```python
from build123d import *

# Parameters (mm, degrees)
ESQUISSE1_W             = 55
ESQUISSE1_H             = 55
BOSS_EXTRU_1_DEPTH      = 5
ESQUISSE2_W             = 30
ESQUISSE2_H             = 15
BOSS_EXTRU_2_DEPTH      = 60
CONG_2_R                = 5
CONG_3_R                = 5
CONG_4_R                = 5
CONG_5_R                = 5
ENL_V_MAT_EXTRU_1_REACH = 7
ESQUISSE3_R             = 1
ESQUISSE4_R             = 0.5
ENL_V_MAT_EXTRU_2_DEPTH = 2


with BuildPart() as part:
    # Esquisse1 → Boss.-Extru.1 (new body)
    with BuildSketch(Plane.XY):
        Rectangle(ESQUISSE1_W, ESQUISSE1_H)
    extrude(amount=BOSS_EXTRU_1_DEPTH)

    # Esquisse2 → Boss.-Extru.2 (add)
    with BuildSketch(Plane.XY.offset(5)):
        Rectangle(ESQUISSE2_W, ESQUISSE2_H)
    extrude(amount=BOSS_EXTRU_2_DEPTH)

    # Congé2
    cong_2_edges = [part.edges().sort_by_distance(p)[0] for p in [
        (-15, -7.5, 35),
    ]]
    fillet(cong_2_edges, radius=CONG_2_R)

    # Congé3
    cong_3_edges = [part.edges().sort_by_distance(p)[0] for p in [
        (15, 7.5, 35),
    ]]
    fillet(cong_3_edges, radius=CONG_3_R)

    # Congé4
    cong_4_edges = [part.edges().sort_by_distance(p)[0] for p in [
        (15, -7.5, 35),
    ]]
    fillet(cong_4_edges, radius=CONG_4_R)

    # Congé5
    cong_5_edges = [part.edges().sort_by_distance(p)[0] for p in [
        (-15, 7.5, 35),
    ]]
    fillet(cong_5_edges, radius=CONG_5_R)

    # Esquisse3 → Enlèv. mat.-Extru.1 (cut, up to next)
    with BuildSketch(Plane.XY.offset(5), mode=Mode.PRIVATE) as enl_v_mat_extru_1_sk1:
        with Locations((17.5, 17.5)):
            Circle(ESQUISSE3_R)
    enl_v_mat_extru_1_tool1 = extrude(enl_v_mat_extru_1_sk1.sketch, amount=-ENL_V_MAT_EXTRU_1_REACH, mode=Mode.PRIVATE) & part.part
    add(enl_v_mat_extru_1_tool1.solids().sort_by_distance((17.5, 17.5, 5))[0], mode=Mode.SUBTRACT)
    # Esquisse3 → Enlèv. mat.-Extru.1 (cut, up to next)
    with BuildSketch(Plane.XY.offset(5), mode=Mode.PRIVATE) as enl_v_mat_extru_1_sk2:
        with Locations((-17.5, 17.5)):
            Circle(ESQUISSE3_R)
    enl_v_mat_extru_1_tool2 = extrude(enl_v_mat_extru_1_sk2.sketch, amount=-ENL_V_MAT_EXTRU_1_REACH, mode=Mode.PRIVATE) & part.part
    add(enl_v_mat_extru_1_tool2.solids().sort_by_distance((-17.5, 17.5, 5))[0], mode=Mode.SUBTRACT)
    # Esquisse3 → Enlèv. mat.-Extru.1 (cut, up to next)
    with BuildSketch(Plane.XY.offset(5), mode=Mode.PRIVATE) as enl_v_mat_extru_1_sk3:
        with Locations((-17.5, -17.5)):
            Circle(ESQUISSE3_R)
    enl_v_mat_extru_1_tool3 = extrude(enl_v_mat_extru_1_sk3.sketch, amount=-ENL_V_MAT_EXTRU_1_REACH, mode=Mode.PRIVATE) & part.part
    add(enl_v_mat_extru_1_tool3.solids().sort_by_distance((-17.5, -17.5, 5))[0], mode=Mode.SUBTRACT)
    # Esquisse3 → Enlèv. mat.-Extru.1 (cut, up to next)
    with BuildSketch(Plane.XY.offset(5), mode=Mode.PRIVATE) as enl_v_mat_extru_1_sk4:
        with Locations((17.5, -17.5)):
            Circle(ESQUISSE3_R)
    enl_v_mat_extru_1_tool4 = extrude(enl_v_mat_extru_1_sk4.sketch, amount=-ENL_V_MAT_EXTRU_1_REACH, mode=Mode.PRIVATE) & part.part
    add(enl_v_mat_extru_1_tool4.solids().sort_by_distance((17.5, -17.5, 5))[0], mode=Mode.SUBTRACT)

    # Esquisse4 → Enlèv. mat.-Extru.2 (cut)
    with BuildSketch(Plane.XY.offset(65)):
        with Locations((10, -2.5)):
            Circle(ESQUISSE4_R)
        with Locations((10, 2.5)):
            Circle(ESQUISSE4_R)
        with Locations((-10, 2.5)):
            Circle(ESQUISSE4_R)
        with Locations((-10, -2.5)):
            Circle(ESQUISSE4_R)
    extrude(amount=-ENL_V_MAT_EXTRU_2_DEPTH, mode=Mode.SUBTRACT)


solid = part.part
```
Part model, mm, in its own coordinate system. A direction names the side the tool comes from. Coordinates: 2 decimals unless noted, no trailing zeros. Loops run counter-clockwise (first coordinate to the right, second up) from the corner with the lowest first, then second, coordinate; pieces in that order, holes last. Notation, with made-up numbers: (63.5, 43) - (67.5, 43) arc R21 ccw to (67.5, 76) - close; hole circle Ø3 at (65.25, 43.25). An arc over 180 degrees is marked (long way). Write item = value, one per line. Start each with the question number.
Item 1: Cut at D-D, the plane y = -12.5. Give the cut face in (x, z), and give its area (3 significant figures).
Item 2: Cut at A-A, the plane x = 17.5. Give the cut face in (y, z), and give its area (3 significant figures).
Item 3: Flat gauge pins, fed straight in: pin 1 Ø10 at (y, z) = (5.5, 45.5) entering from -X; pin 2 Ø2.5 at (y, z) = (-1, 39) entering from +X; pin 3 Ø0.8 at (x, y) = (10, -2.5) entering from +Z. Where does each tip first touch, or does it go through?
Item 4: 3-axis set-ups, long thin cutter, end or side, ignore diameter. For faces 5 (the cylindrical face through (-13.5, -6.07, 35.42)), 6 (the cylindrical face through (13.57, -6, 35.42)), 7 (the flat face through (0, -7.5, 35)), 8 (the flat face through (15, 0, 35)), 9 (the flat face through (-15, 0, 35)): which of +Z, -Z, +X, -X, +Y, -Y reach the whole face in a straight line?
Item 5: Wall check: L1, parallel to Y at x = 17.5, z = 2.95; L2, parallel to Y at x = 10, z = 64.05; L3, parallel to X at y = 17, z = 3. Give the ranges that are in metal, low to high. Write a range as from..to.
Item 6: Mould opens along Y. For faces 1 (the flat face through (0, 0, 65)), 2 (the cylindrical face through (17.96, 16.61, 2.54)), 3 (the cylindrical face through (-17.04, 16.61, 2.54)), 4 (the cylindrical face through (-13.5, 6.07, 35.42)) say: released by +Y, released by -Y, zero draft, split by the parting line, or undercut.
Item 7: Cut at B-B, the plane z = 57. Give the cut face in (x, y), and give its area (3 significant figures).
The answers:
q1.outline = (-27.5, 0) - (27.5, 0) - (27.5, 5) - (-27.5, 5) - close
q1.area = 275 mm2
q2.outline = (-27.5, 0) - (-18.5, 0) - (-18.5, 5) - (-27.5, 5) - close; (-16.5, 0) - (16.5, 0) - (16.5, 5) - (-16.5, 5) - close; (18.5, 0) - (27.5, 0) - (27.5, 5) - (18.5, 5) - close
q2.area = 255 mm2
q3.pin_1 = -15
q3.pin_2 = 15
q3.pin_3 = 63
q4.face_5 = +Z, -X, -Y
q4.face_6 = +Z, +X, -Y
q4.face_7 = +Z, +X, -X, -Y
q4.face_8 = +Z, +X, +Y, -Y
q4.face_9 = +Z, -X, +Y, -Y
q5.L1 = -27.5..-18.5, -16.5..16.5, 18.5..27.5
q5.L2 = -7.5..-3, -2..2, 3..7.5
q5.L3 = -27.5..-18.37, -16.63..16.63, 18.37..27.5
q6.face_1 = zero draft
q6.face_2 = undercut
q6.face_3 = undercut
q6.face_4 = released by +Y
q7.outline = (-15, -2.5) arc R5 ccw to (-10, -7.5) - (10, -7.5) arc R5 ccw to (15, -2.5) - (15, 2.5) arc R5 ccw to (10, 7.5) - (-10, 7.5) arc R5 ccw to (-15, 2.5) - close
q7.area = 429 mm2
